Geometry: see drawing. Coordinates: mm, zero at the bounding-box minimum. Give positions to 0.01 mm unless a question says otherwise; leave off trailing zeros. Order: outer loops, then holes, each group sorted by start corner. A loop starts at its lowest first (then second) coordinate and runs counter-clockwise, first axis right, second up. Notation, with made-up numbers: M -12.75,-32 L 40.25,-32 A27 cw 40.25,-15 Z; hole C 47,69 d8. An arc over 180 degrees is marked long. Answer as a JSON object with one key per item and string values. Group by question number.
1. Section query A-A (y = 52). Output: boundary loops of the cut face in (x, z), plus the area to 3 significant figures.
2. Pull-direction query (Y, two-part tool) for the marked faces 1 and 2; classes: +Y half, -Y half, draft (parallel to the pull), parting line (faces both ways), or undercut.
3. Section query B-B (x = 52). Output: boundary loops of the cut face in (y, z), plus the area to 3 significant figures.
4. Pin query (flat end, axial travel): P1, Ø10, axis at y = 16, z = 18, coming from the +X side; P2, Ø3, axis at y = 93.5, z = 22, coming from the +X side; P3, Ø2, axis at x = 83.5, z = 19, coming from the +Y side; P4, Ø1, axis at x = 11.5, y = 80, coming from the +Z side. Return the tip coordinate at first contact, or that it passes through.
5. Section query C-C (z = 16). Output: boundary loops of the cut face in (x, y).
6. Section query D-D (z = 5.5). Output: boundary loops of the cut face in (x, y).
7. Material intervals for L1, parallel to Y at x = 52, z = 51.4; L2, parallel to Y at x = 52, z = 34; L3, parallel to X at y = 12, z = 34.5, sorted ascending. Write a range as [from, to].
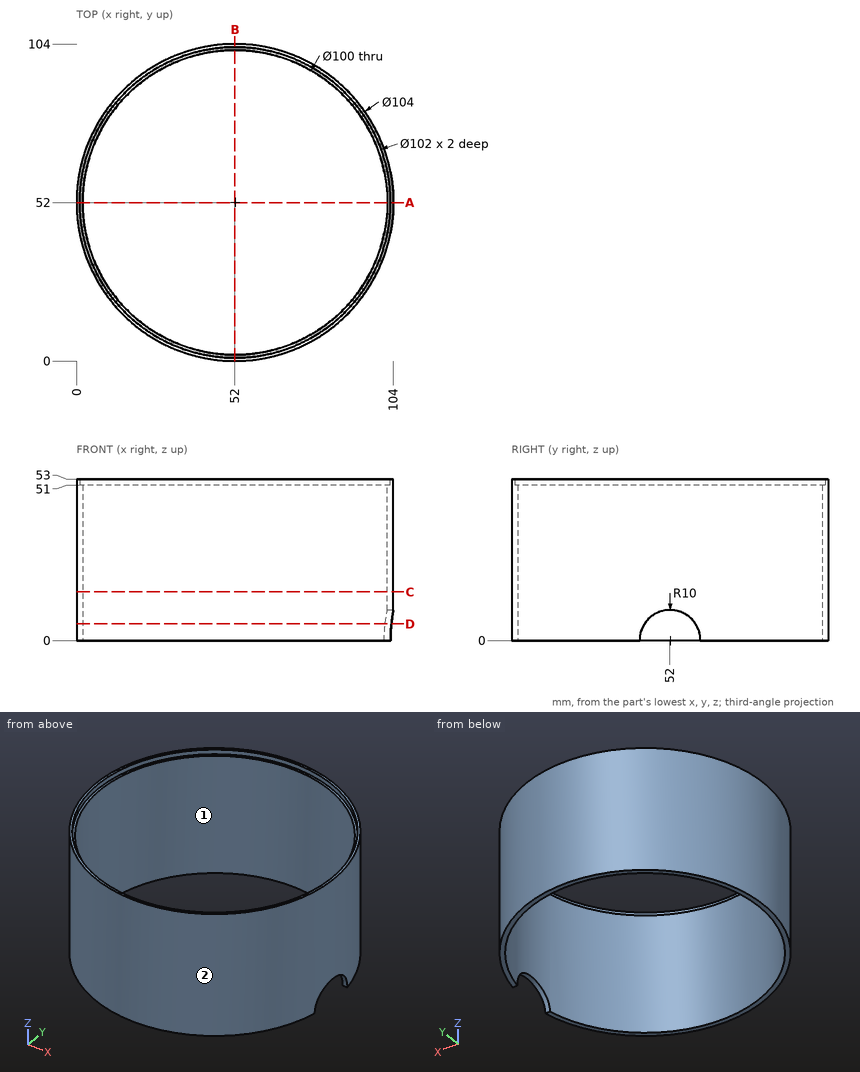
Answer sheet:
{
 "1": {"outline": "M 0,0 L 2,0 L 2,51 L 1,51 L 1,53 L 0,53 Z; M 102,10 L 104,10 L 104,53 L 103,53 L 103,51 L 102,51 Z", "area": "188 mm^2"},
 "2": {"face 1": "undercut", "face 2": "parting line"},
 "3": {"outline": "M 0,0 L 2,0 L 2,51 L 1,51 L 1,53 L 0,53 Z; M 102,0 L 104,0 L 104,53 L 103,53 L 103,51 L 102,51 Z", "area": "208 mm^2"},
 "4": {"P1": "x = 93.75", "P2": "x = 85.23", "P3": "y = 94.12", "P4": "through"},
 "5": {"outline": "C 52,52 d104; hole C 52,52 d100"},
 "6": {"outline": "M 101.3,43.65 A50 cw long 101.3,60.35 L 103.32,60.35 A52 ccw long 103.32,43.65 Z"},
 "7": {"L1": "[0, 1], [103, 104]", "L2": "[0, 2], [102, 104]", "L3": "[18.77, 22], [82, 85.23]"}
}
